from build123d import *

# Parameters (mm, degrees)
SKETCH_1_W          = 200
SKETCH_1_H          = 80
EXTRUDE_1_DEPTH     = 10
SKETCH_3_W          = 50
SKETCH_3_H          = 150
EXTRUDE_2_DEPTH     = 10
SKETCH_5_R          = 1.7
SKETCH_5_R_2        = 7.5
CUT_EXTRUDE_3_DEPTH = 10
SKETCH_6_R          = 1.7
CUT_EXTRUDE_4_DEPTH = 10
SKETCH_7_R          = 3.7
CUT_EXTRUDE_5_DEPTH = 4.5


with BuildPart() as part:
    # 草图1 → 凸台-拉伸1 (new body)
    with BuildSketch(Plane(origin=(0, 0, 0), x_dir=(1, 0, 0), z_dir=(0, 1, 0))):
        Rectangle(SKETCH_1_W, SKETCH_1_H)
    extrude(amount=EXTRUDE_1_DEPTH)

    # 草图3 → 凸台-拉伸2 (add)
    with BuildSketch(Plane(origin=(0, 10, 0), x_dir=(1, 0, 0), z_dir=(0, 1, 0))):
        Rectangle(SKETCH_3_W, SKETCH_3_H)
    extrude(amount=-EXTRUDE_2_DEPTH)

    # 草图5 → 切除-拉伸3 (cut)
    with BuildSketch(Plane(origin=(0, 10, 0), x_dir=(1, 0, 0), z_dir=(0, 1, 0))):
        with Locations((13.435028843, 13.435028843)):
            Circle(SKETCH_5_R)
        with Locations((13.435028843, -13.435028843)):
            Circle(SKETCH_5_R)
        with Locations((-13.435028843, -13.435028843)):
            Circle(SKETCH_5_R)
        with Locations((-13.435028843, 13.435028843)):
            Circle(SKETCH_5_R)
        Circle(SKETCH_5_R_2)
    extrude(amount=-CUT_EXTRUDE_3_DEPTH, mode=Mode.SUBTRACT)

    # 草图6 → 切除-拉伸4 (cut)
    with BuildSketch(Plane(origin=(0, 10, 0), x_dir=(1, 0, 0), z_dir=(0, 1, 0))):
        with Locations((0, 50)):
            Circle(SKETCH_6_R)
        with Locations((35.355339059, 35.355339059)):
            Circle(SKETCH_6_R)
        with Locations((50, 0)):
            Circle(SKETCH_6_R)
        with Locations((35.355339059, -35.355339059)):
            Circle(SKETCH_6_R)
        with Locations((0, -50)):
            Circle(SKETCH_6_R)
        with Locations((-35.355339059, -35.355339059)):
            Circle(SKETCH_6_R)
        with Locations((-50, 0)):
            Circle(SKETCH_6_R)
        with Locations((-35.355339059, 35.355339059)):
            Circle(SKETCH_6_R)
    extrude(amount=-CUT_EXTRUDE_4_DEPTH, mode=Mode.SUBTRACT)

    # 草图7 → 切除-拉伸5 (cut)
    with BuildSketch(Plane(origin=(0, 10, 0), x_dir=(1, 0, 0), z_dir=(0, 1, 0))):
        with Locations((0, 50)):
            Circle(SKETCH_7_R)
        with Locations((13.435028843, 13.435028843)):
            Circle(SKETCH_7_R)
        with Locations((35.355339059, 35.355339059)):
            Circle(SKETCH_7_R)
        with Locations((50, 0)):
            Circle(SKETCH_7_R)
        with Locations((35.355339059, -35.355339059)):
            Circle(SKETCH_7_R)
        with Locations((0, -50)):
            Circle(SKETCH_7_R)
        with Locations((-35.355339059, -35.355339059)):
            Circle(SKETCH_7_R)
        with Locations((-50, 0)):
            Circle(SKETCH_7_R)
        with Locations((-35.355339059, 35.355339059)):
            Circle(SKETCH_7_R)
        with Locations((13.435028843, -13.435028843)):
            Circle(SKETCH_7_R)
        with Locations((-13.435028843, -13.435028843)):
            Circle(SKETCH_7_R)
        with Locations((-13.435028843, 13.435028843)):
            Circle(SKETCH_7_R)
    extrude(amount=-CUT_EXTRUDE_5_DEPTH, mode=Mode.SUBTRACT)


solid = part.part
Verification items for the finished model (mm, model axes). A direction names the side the tool comes from. Coordinates: 2 decimals unless noted, no trailing zeros. Order: outer loops, then holes, each group sorted by start corner. A loop starts at its lowest first (then second) coordinate and runs counter-clockwise, first axis right, second up. Notation, with made-up numbers: M -11,10.25 L 33,10.25 A14 ccw 33,24.25 Z; hole C 78,47.5 d10. An arc over 180 degrees is marked long. Return JSON: item names as keys, results as strings.
1) Cross-section at B-B, the plane z = -65. Record the boundary of the cut face in (x, y), and give its area (3 significant figures).
Answer list:
{"outline": "M -25,0 L 25,0 L 25,10 L -25,10 Z", "area": "500 mm2"}
2) Release check for a two-part mould opening along X. For faces 1 (the flat face through (-25, 5, 58)), 2 (the flat face through (14.21, 5.5, -15.13)), 3 (the flat face through (0, 5, -75)) record: +X half, -X half, draft (parallel to the pull), parting line (faces both ways), or undercut.
Answer list:
{"face 1": "-X half", "face 2": "undercut", "face 3": "draft"}
3) Cross-section at A-A, the plane y = 7.75. Count the separate pieces of the cut face and the enclosed holes in it, and give its area (3 significant figures).
Answer list:
{"separate pieces": "1", "enclosed holes": "13", "area": "18,800 mm2"}
4) Access from +Z, -Z, +X, -X, +Y, -Y to the whole of each face (thin tool, end or side, straight path). Record for faces 4 (the cylindrical face through (-14.237, 7.781, 17.047)), 5 (the flat face through (25, 5, -57)), 6 (the flat face through (-25, 5, -57)).
Answer list:
{"face 4": "+Y", "face 5": "-Z, +X, +Y, -Y", "face 6": "-Z, -X, +Y, -Y"}
5) Gauge pin test, flat ends, axial feed: pin 1 (5.5 mm diameter, centred on x = -35.36, z = -35.36, fed in from +Y); pin 2 (1 mm diameter, centred on x = -37.5, y = 1.5, fed in from -Z); pin 3 (3 mm diameter, centred on x = 71, y = 6.5, fed in from +Z). Record the tip position at first contact, or that the pin passes through.
Answer list:
{"pin 1": "y = 5.5", "pin 2": "z = -40", "pin 3": "z = 40"}
6) Thickness scan on L1, parallel to Z at x = 0, y = 3.5; L2, parallel to X at y = 2.3, z = 0; L3, parallel to X at y = 7.3, z = 0. Record the ranges inside material, lowest first. Write a range as [from, to].
Answer list:
{"L1": "[-75, -51.7], [-48.3, -7.5], [7.5, 48.3], [51.7, 75]", "L2": "[-100, -51.7], [-48.3, -7.5], [7.5, 48.3], [51.7, 100]", "L3": "[-100, -53.7], [-46.3, -7.5], [7.5, 46.3], [53.7, 100]"}
